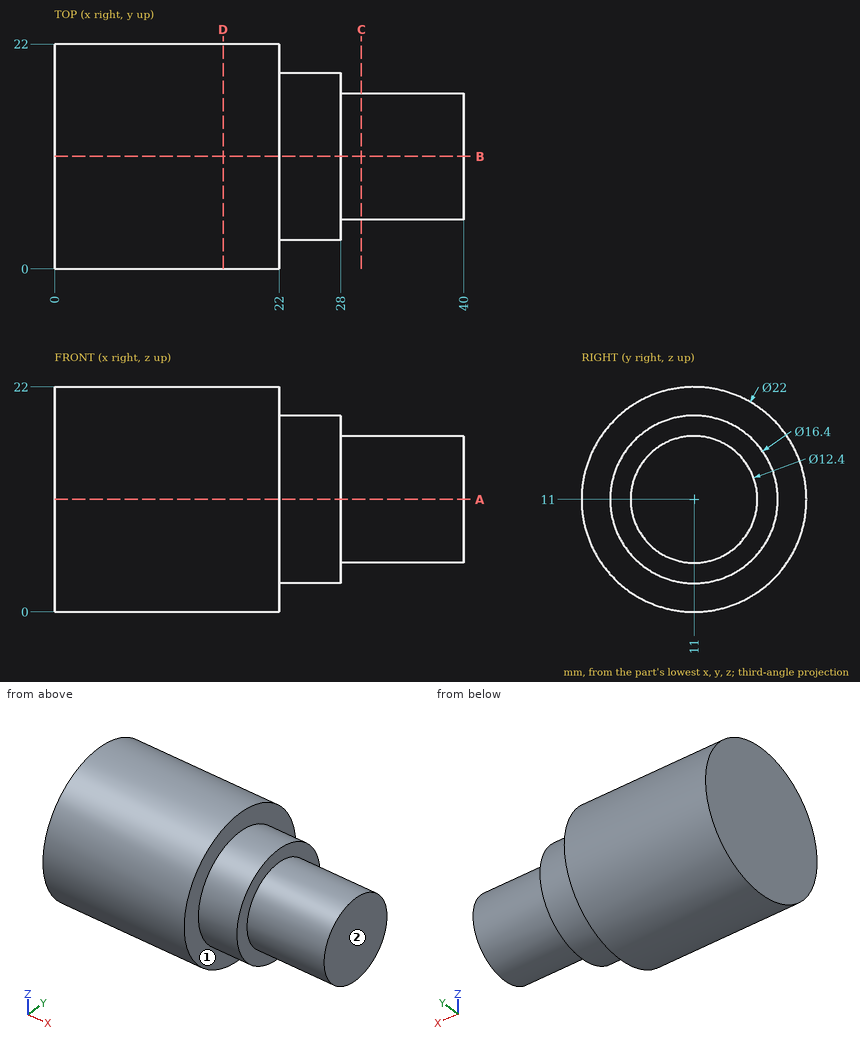
Print and shaded views of the part. All mm, measured from the part's lowest x, y and z. A direction names the side the tool comes from. Give positions to 0.01 mm unless a question says otherwise; leave off trailing zeros. Loops run counter-clockwise (first coordinate to the right, second up) from the corner with the lowest first, then second, coordinate; pieces in that order, holes last.
1) Saw through at D-D (x = 16.5). Write the cut outline in (y, z), plus the area to 3 significant figures.
2) Saw through at A-A (z = 11). Write the cut outline in (x, y).
3) Saw through at C-C (x = 30). Write the cut outline in (y, z), plus the area to 3 significant figures.
4) Tool access for the marked faces 1 and 2: list every direction of +Z, -Z, +X, -X, +Y, -Y with a clear straight run to the whole face (end or side of a thin tool).
5) Wall check: line 1 (X direction, y = 18.75, z = 5.5); line 2 (X direction, y = 18.25, z = 12.25); line 3 (Z direction, x = 31, y = 11). Give the ranges that are in metal, low to high.
6) Flat gauge pins, fed straight in: pin 1 Ø5 at (y, z) = (18, 6) entering from -X; pin 2 Ø1 at (x, z) = (16.5, 2.5) entering from -Y; pin 3 Ø4 at (x, y) = (10.5, 4.5) entering from +Z; pin 4 Ø3 at (x, y) = (8, 8.5) entering from +Z. Where does each tip first touch, or does it go through?
Answer block:
1. outline: circle Ø22 at (11, 11)
1. area: 380 mm2
2. outline: (0, 0) - (22, 0) - (22, 2.8) - (28, 2.8) - (28, 4.8) - (40, 4.8) - (40, 17.2) - (28, 17.2) - (28, 19.2) - (22, 19.2) - (22, 22) - (0, 22) - close
3. outline: circle Ø12.4 at (11, 11)
3. area: 121 mm2
4. face 1: +X
4. face 2: +Z, -Z, +X, +Y, -Y
5. line 1: x = 0 to 22
5. line 2: x = 0 to 28
5. line 3: z = 4.8 to 17.2
6. pin 1: stops at x = 0
6. pin 2: stops at y = 3.45
6. pin 3: stops at z = 21.04
6. pin 4: stops at z = 21.95
